Study the drawing (mm; zero at the part's minimum x, y, z) and answer. A direction names the side the tool comes from. Round coordinates to 2 decimals unless told otherwise and drop trailing zeros. Write each loop counter-clockwise with the first axis right and the second up, starting at its lowest first coordinate (ties: lowest second). Pieces come first, ordered by that corner, then holes. Notation, with made-up numbers: (12, 3) - (26, 3) arc R27 ccw to (26, 20) - close; hole circle Ø4 at (-34, 32.5). An arc over 180 degrees is marked (long way). Return JSON: item names as keys, results as strings. Group by question number.
(1) Section B-B, the plane y = 6.25 is taken. Give the number of separate pieces and of enclosed holes in the cut face, then the cut area to 3 significant figures.
(2) Section D-D, the plane y = 2.25 is taken. Write down the section's boundary in (x, z) (1 decimal), then the cut area to 3 significant figures.
(3) Find the intervals of material crossed by line 1 along X through (y, z) = (19.25, 13) (1 decimal); line 2 along Y through (x, z) = (8, 8); line 3 along X through (y, z) = (12, 7) (1 decimal), in increasing order. Write a range as [from, to].
(4) Section A-A, the plane z = 2 is taken. Write down the section's boundary in (x, y) (1 decimal).
(5) Determine the mould class of the marked faces 1, 2, 3 and 4 for opening direction Z: +Z half, -Z half, draft (parallel to the pull), parting line (faces both ways), or undercut.
(6) Section C-C, the plane z = 28.5 is taken. Write down the section's boundary in (x, y) (1 decimal).
(7) Each of these flat-tipped pins is pushed along its axis until it touches: pin 1 (4 mm diameter, centred on x = 12.04, z = 3.28, fed in from +Y); pin 2 (4 mm diameter, centred on y = 18.5, z = 19, fed in from -X); pin 3 (12 mm diameter, centred on y = 8.5, z = 27, fed in from -X) (1 decimal). Where does it stop, or does it pass through?
(8) Which of the six approach directions +Z, -Z, +X, -X, +Y, -Y give full straight-line access (tool end or side, diameter ignored) to the marked faces 5, 6 and 7?
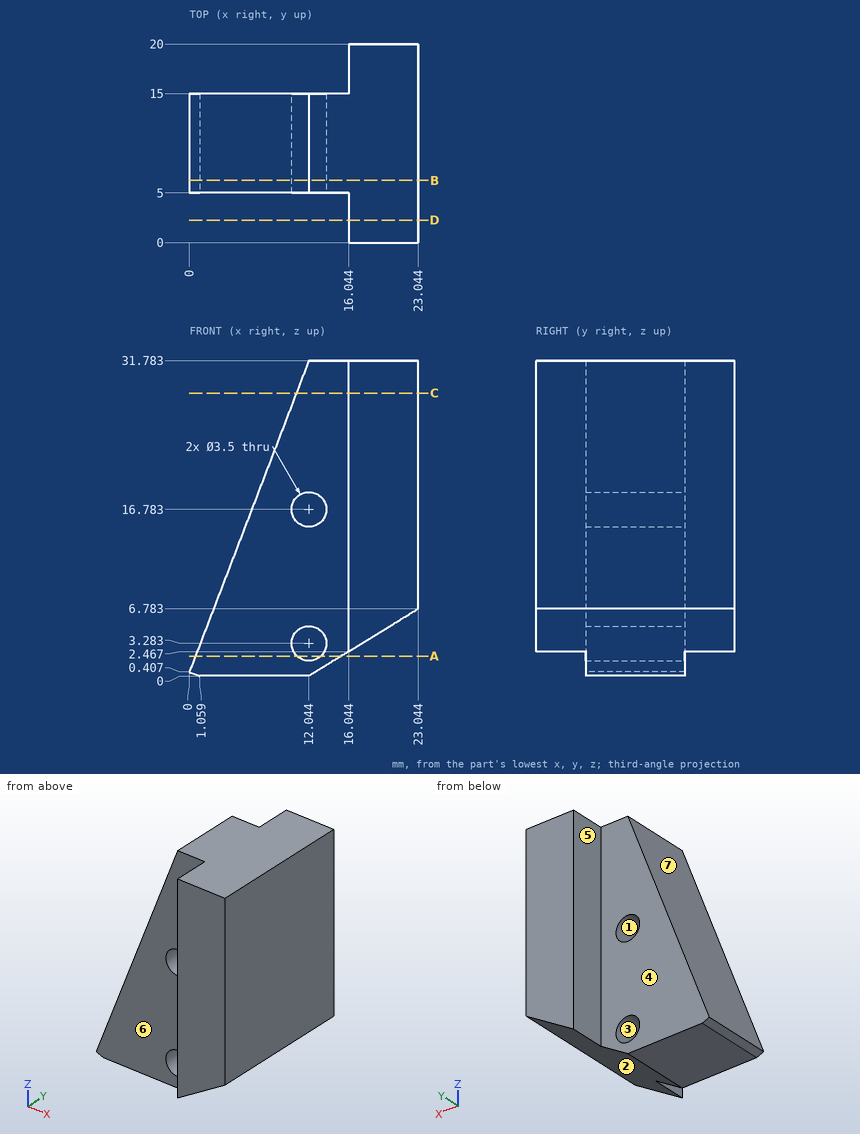
Working result:
{
 "1": {"separate pieces": "1", "enclosed holes": "2", "area": "487 mm^2"},
 "2": {"outline": "(16, 2.5) - (23, 6.8) - (23, 31.8) - (16, 31.8) - close", "area": "190 mm^2"},
 "3": {"line 1": "x = [16, 23]", "line 2": "y = [5, 15]", "line 3": "x = [2.5, 23]"},
 "4": {"outline": "(0.6, 5) - (10.9, 5) - (10.9, 15) - (0.6, 15) - close; (13.2, 5) - (15.3, 5) - (15.3, 15) - (13.2, 15) - close"},
 "5": {"face 1": "undercut", "face 2": "-Z half", "face 3": "undercut", "face 4": "draft"},
 "6": {"outline": "(10.8, 5) - (16, 5) - (16, 0) - (23, 0) - (23, 20) - (16, 20) - (16, 15) - (10.8, 15) - close"},
 "7": {"pin 1": "stops at y = 15", "pin 2": "stops at x = 16.04", "pin 3": "stops at x = 7.9"},
 "8": {"face 5": "+Z, -Z, -X, +Y", "face 6": "+Z, -Z, -X, -Y", "face 7": "+Z, -X, +Y, -Y"}
}
